Source: CAD feature listing. Evaluate the final solid. Frame: model axes, mm. A direction names the side the tool comes from. Give positions to 0.01 mm unless a question says otherwise; leave off trailing zeros. Write each loop counter-clockwise with the first axis right and the second up, starting at its lowest first coordinate (ties: lowest second). Pieces come first, ordered by that corner, then holes. Notation, with made-up numbers: M 20.25,-26.75 L 69.25,-26.75 A34 cw 69.25,11.25 Z; hole C 67,1 d2. An arc over 180 degrees is marked long. Answer as a JSON object with one key per item and string values. Group by question number.
Autodesk Inventor part; units mm, degrees
sketch "スケッチ1" plane through (0, 0, 0) normal (0, 0, 1) x (1, 0, 0)
  circle A0 centre (0, 0) radius 17.5
  dimension "d0" = 35
extrude "押し出し1" add sketch "スケッチ1" along normal blind 20
sketch "スケッチ2" plane through (0, 0, 20) normal (0, 0, 1) x (1, 0, 0)
  circle A0 centre (0, 0) radius 25
  dimension "d3" = 50
extrude "押し出し2" add sketch "スケッチ2" along normal blind 70
sketch "スケッチ3" plane through (0, 0, 90) normal (0, 0, 1) x (1, 0, 0)
  circle A0 centre (0, 0) radius 17.5
  dimension "d6" = 35
extrude "押し出し3" add sketch "スケッチ3" along normal blind 20
sketch "スケッチ4" plane through (0, 0, 0) normal (1, 0, 0) x (0, 1, 0)
  point P0 (0, 0)
ref_plane "作業平面2" through (0, 0, 55) normal (0, 0, 1) x (1, 0, 0)
ref_plane "作業平面1" through (0, 0, 110) normal (0, 0, 1) x (1, 0, 0)
ref_plane "作業平面3" through (0, 25, 0) normal (0, 1, 0) x (-1, 0, 0)
sketch "スケッチ8" plane through (0, 25, 0) normal (0, 1, 0) x (-1, 0, 0)
  line L0 (-7, 25) -> (7, 25)
  line L1 (0, 25) -> (0, 32)
  line L2 (0, 25) -> (7, 25) construction
  line L3 (-7, 25) -> (-7, 85)
  arc A0 (-7, 32) -> (7, 32) centre (0, 32) ccw
  line L4 (7, 85) -> (7, 25)
  line L5 (7, 32) -> (7, 25)
  line L6 (7, 25) -> (0, 25)
  line L7 (-7, 25) -> (-7, 32)
  line L8 (0, 25) -> (-7, 25)
  line L9 (7, 85) -> (-7, 85)
  line L10 (7, 55) -> (-7, 55)
  arc A1 (7, 78) -> (-7, 78) centre (0, 78) ccw
  point P0 (0, 0)
  dimension "d17" = 7
  dimension "d18" = 90
  dimension "d21" = 30
extrude "押し出し5" cut sketch "スケッチ8" against normal blind 5.5 contours A0 L3 L10 L4 | L3 A1 L4 L10
properties part number "shaft1"
(1) Pull-direction query (Z, two-part tool) for faces 4 (the flat face through (-17, -5, 20)), 5 (the cylindrical face through (-13.887, 10.648, 99.86)), 6 (the flat face through (7, 22, 55)); classes: pulls with the +Z half, pulls with the -Z half, needs draft (parallel to the pull), parting line crosses it, or undercut.
(2) Section B-B, the plane y = 0. Return loops of the section in (x, z).
(3) Ray query, L1, parallel to Z at x = -19, y = -5; L2, parallel to X at y = 1, z = 87.5; L3, parallel to Y at x = -1, z = 65. Return the intervals inside material, ascending. Write a range as [from, to].
(4) Section D-D, the plane y = 14.5. Return loops of the section in (x, z), plus the area to 4 significant figures.
(5) Section A-A, the plane x = 0. Return loops of the section in (y, z), plus the area to 3 significant figures.
(6) Access query for faces 1 (the cylindrical face through (0, 22, 25)), 2 (the flat face through (-17, -5, 90)), 3 (the cylindrical face through (-13.887, 10.648, 9.86)). Directions: +Z, -Z, +X, -X, +Y, -Y. A direction counts if a zero-diameter tool reaches every point of the face in a straight line with its end or side. Return the directions, or none.
(7) Contact query for flat-ended pins moving along their axis: pin 1 Ø1 at (x, z) = (-11.5, 45.5) entering from +Y; pin 2 Ø5 at (x, z) = (1, 42.5) entering from +Y; pin 3 Ø10 at (x, z) = (-12, 57.5) entering from -Y. Output: stop coordinate, or through.
(8) Section C-C, the plane z = 23. Return loops of the section in (x, y), plus the area to 3 significant figures.
Reported:
{
 "1": {"face 4": "pulls with the -Z half", "face 5": "needs draft", "face 6": "undercut"},
 "2": {"outline": "M -25,20 L -17.5,20 L -17.5,0 L 17.5,0 L 17.5,20 L 25,20 L 25,90 L 17.5,90 L 17.5,110 L -17.5,110 L -17.5,90 L -25,90 Z"},
 "3": {"L1": "z = [20, 90]", "L2": "x = [-24.98, 24.98]", "L3": "y = [-24.98, 19.5]"},
 "4": {"outline": "M -20.37,20 L -9.8,20 L -9.8,0 L 9.8,0 L 9.8,20 L 20.37,20 L 20.37,90 L 9.8,90 L 9.8,110 L -9.8,110 L -9.8,90 L -20.37,90 Z", "area": "3,635 mm2"},
 "5": {"outline": "M -25,20 L -17.5,20 L -17.5,0 L 17.5,0 L 17.5,20 L 25,20 L 25,25 L 19.5,25 L 19.5,85 L 25,85 L 25,90 L 17.5,90 L 17.5,110 L -17.5,110 L -17.5,90 L -25,90 Z", "area": "4,570 mm2"},
 "6": {"face 1": "+Y", "face 2": "+Z", "face 3": "-Z"},
 "7": {"pin 1": "stops at y = 22.45", "pin 2": "stops at y = 19.5", "pin 3": "stops at y = -24"},
 "8": {"outline": "C 0,0 d50", "area": "1,960 mm2"}
}
